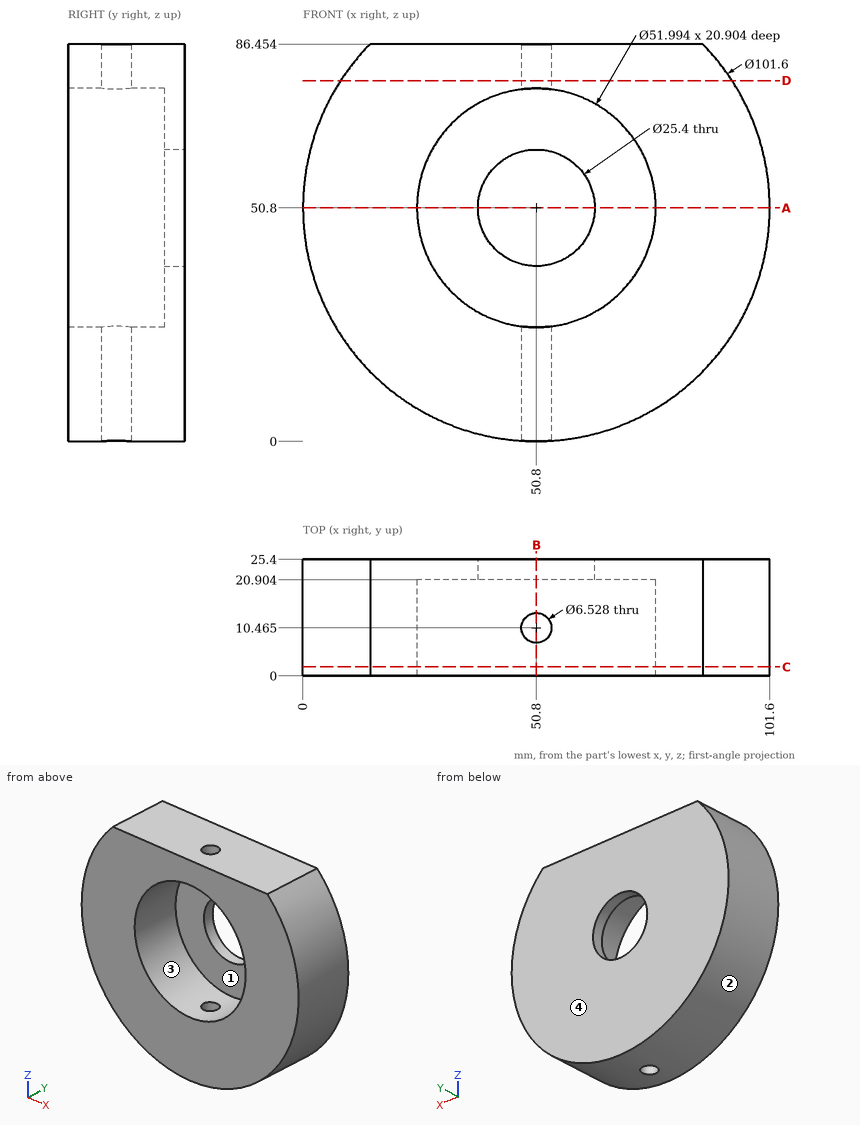
Geometry: see drawing. Coordinates: mm, zero at the bounding-box minimum. Coordinates: 2 decimals unless noted, no trailing zeros. Write each loop counter-clockwise with the first axis right and the second up, starting at its lowest first coordinate (ties: lowest second). Pieces come first, ordered by that corner, then holes. Notation, with made-up numbers: M -9.5,29.5 L 8.5,29.5 A7 cw 8.5,36.5 Z; hole C -19.5,64.25 d5. An arc over 180 degrees is marked long. Use CSV: the item, a comma, the result in double quotes. Start each with the question number.
1. Ray query, probe 1 along Z at (x, y) = (50.8, 22.75) (1 decimal); probe 2 along X at (y, z) = (8.5, 4.5) (1 decimal); probe 3 along X at (y, z) = (16.75, 57.5) (1 decimal). Return the intervals inside material, ascending.
2. Cut plane B-B on x = 50.8. Return the cut outline in (y, z) (1 decimal).
3. Cut plane D-D on z = 78.5. Return the cut outline in (x, y) (1 decimal), plus the area to 3 significant figures.
4. Mould query, pull axis X, two halves, no side actions, for the marked faces 1, 2, 3 and 4. Classes: pulls with the +X half, pulls with the -X half, needs draft (parallel to the pull), parting line crosses it, or undercut.
5. Cut plane A-A on z = 50.8. Return the cut outline in (x, y) (1 decimal), plus the area to 3 significant figures.
6. First-contact query: P1, Ø4, axis at y = 16, z = 38.5, coming from the +X side (1 decimal); P2, Ø8, axis at y = 15, z = 33.5, coming from the -X side; P3, Ø10, axis at y = 21, z = 15, coming from the +X side; P4, Ø23, axis at x = 50.8, z = 50.8, coming from the +Y side. Flat tips, straight axial feed; report the tip coordinate or a pass-through.
7. Cut plane C-C on y = 2. Return the cut outline in (x, z) (1 decimal).
Entries:
1,probe 1,"0 to 38.1, 63.5 to 86.5"
1,probe 2,"29.9 to 48.2, 53.4 to 71.7"
1,probe 3,"0.4 to 25.7, 75.9 to 101.2"
2,outline,"M 0,0 L 7.2,0 L 7.2,24.8 L 0,24.8 Z; M 0,76.8 L 7.2,76.8 L 7.2,86.5 L 0,86.5 Z; M 13.7,0 L 25.4,0 L 25.4,38.1 L 20.9,38.1 L 20.9,24.8 L 13.7,24.8 Z; M 13.7,76.8 L 20.9,76.8 L 20.9,63.5 L 25.4,63.5 L 25.4,86.5 L 13.7,86.5 Z"
3,outline,"M 8.2,0 L 93.4,0 L 93.4,25.4 L 8.2,25.4 Z; hole C 50.8,10.5 d6.5"
3,area,"2,130 mm²"
4,face 1,"undercut"
4,face 2,"parting line crosses it"
4,face 3,"undercut"
4,face 4,"needs draft"
5,outline,"M 0,0 L 24.8,0 L 24.8,20.9 L 38.1,20.9 L 38.1,25.4 L 0,25.4 Z; M 63.5,20.9 L 76.8,20.9 L 76.8,0 L 101.6,0 L 101.6,25.4 L 63.5,25.4 Z"
5,area,"1,380 mm²"
6,P1,"x = 100.5"
6,P2,"x = 1.77"
6,P3,"x = 91.2"
6,P4,"through"
7,outline,"M 14.6,86.5 A50.8 ccw long 87,86.5 Z; hole C 50.8,50.8 d52"
